```python
from build123d import *

# Parameters (mm, degrees)
SKETCH3_W               = 159.804878049
SKETCH3_H               = 120
BOSS_EXTRUDE1_DEPTH     = 10
CUT_EXTRUDE1_DEPTH      = 20
CUT_EXTRUDE3_DEPTH      = 10
CUT_EXTRUDE3_DEPTH_BACK = 16
SKETCH5_R               = 3
CUT_EXTRUDE6_DEPTH      = 10
SKETCH8_R               = 4.027386095
SKETCH8_R_2             = 4.205627654
SKETCH8_R_3             = 4.039456984
SKETCH8_R_4             = 4.036176238
BOSS_EXTRUDE3_DEPTH     = 5
SKETCH9_W               = 33.196532324
SKETCH9_H               = 25.056213838
SKETCH9_R               = 4.18060077
SKETCH9_R_2             = 4.080354001
SKETCH9_R_3             = 4.086165431
SKETCH9_R_4             = 4.036615778
BOSS_EXTRUDE4_DEPTH     = 5


with BuildPart() as part:
    # Sketch3 → Boss-Extrude1 (new body)
    with BuildSketch(Plane(origin=(0, 0, 0), x_dir=(1, 0, 0), z_dir=(0, 1, 0))):
        with Locations((34.390243903, -22.243902439)):
            Rectangle(SKETCH3_W, SKETCH3_H)
    extrude(amount=BOSS_EXTRUDE1_DEPTH)

    # Sketch4 → Cut-Extrude1 (cut)
    with BuildSketch(Plane(origin=(0, 10, 0), x_dir=(1, 0, 0), z_dir=(0, 1, 0))):
        Polygon((52.048199058, -16.00595694), (52.048199058, -34.721676718), (24.165287655, -34.721676718), (24.165287655, -6.031004918), (52.048199058, -6.031004918), align=None)
    extrude(amount=-CUT_EXTRUDE1_DEPTH, mode=Mode.SUBTRACT)

    # Sketch5 → Cut-Extrude3 (cut, two sides: drawn at the far end of the back side and taken through both)
    with BuildSketch(Plane(origin=(0, 10, 0), x_dir=(1, 0, 0), z_dir=(0, 1, 0)).offset(-CUT_EXTRUDE3_DEPTH_BACK)):
        with Locations(Location((-15.512195122, -22.243902439, 0), (0, 0, 270))):
            Circle(SKETCH5_R)
        with Locations(Location((84.292682927, -22.243902439, 0), (0, 0, 270))):
            Circle(SKETCH5_R)
    extrude(amount=CUT_EXTRUDE3_DEPTH + CUT_EXTRUDE3_DEPTH_BACK, mode=Mode.SUBTRACT)

    # Sketch7 → Cut-Extrude6 (cut)
    with BuildSketch(Plane(origin=(0, 10, 0), x_dir=(1, 0, 0), z_dir=(0, 1, 0))):
        Polygon((-6.403519992, -33.196532324), (0, -33.196532324), (0, 0), (-6.403519992, 0), (-28.646264147, 0), (-28.646264147, -33.196532324), align=None)
        Polygon((70.689603866, -33.196532324), (77.304662661, -33.196532324), (99.548678473, -33.196532324), (99.548678473, 0), (77.304662661, 0), (70.689603866, 0), align=None)
    extrude(amount=-CUT_EXTRUDE6_DEPTH, mode=Mode.SUBTRACT)

    # Sketch8 → Boss-Extrude3 (add)
    with BuildSketch(Plane.ZY):
        Polygon((0, 0), (0, 25.089225982), (33.196532324, 25.089225982), (33.196532324, 22.465752332), (33.196532324, 0), align=None)
        with Locations((4.999328758, 20.009772327)):
            Circle(SKETCH8_R, mode=Mode.SUBTRACT)
        with Locations((27.400871365, 20.009772327)):
            Circle(SKETCH8_R_2, mode=Mode.SUBTRACT)
        with Locations((4.999328758, 4.193672126)):
            Circle(SKETCH8_R_3, mode=Mode.SUBTRACT)
        with Locations((27.400871365, 4.193672126)):
            Circle(SKETCH8_R_4, mode=Mode.SUBTRACT)
    extrude(amount=BOSS_EXTRUDE3_DEPTH)

    # Sketch9 → Boss-Extrude4 (add)
    with BuildSketch(Plane(origin=(70.689603866, 0, 0), x_dir=(0, 0, -1), z_dir=(1, 0, 0))):
        with Locations((-16.598266162, 12.528106919)):
            Rectangle(SKETCH9_W, SKETCH9_H)
        with Locations((-28.524013472, 19.041369902)):
            Circle(SKETCH9_R, mode=Mode.SUBTRACT)
        with Locations((-4.413648361, 19.041369902)):
            Circle(SKETCH9_R_2, mode=Mode.SUBTRACT)
        with Locations((-28.524013472, 4.530421359)):
            Circle(SKETCH9_R_3, mode=Mode.SUBTRACT)
        with Locations((-4.413648361, 4.530421359)):
            Circle(SKETCH9_R_4, mode=Mode.SUBTRACT)
    extrude(amount=BOSS_EXTRUDE4_DEPTH)


solid = part.part
```
Can you work these out from the model? Positions are in its coordinate system, mm. A direction names the side the tool comes from. Coordinates: 2 decimals unless noted, no trailing zeros. Order: outer loops, then holes, each group sorted by start corner. A loop starts at its lowest first (then second) coordinate and runs counter-clockwise, first axis right, second up.
1. Thinking about a two-plate mould opening in Z: for faces 1 (the face through (-45.512, 5, 23)), 2 (the face through (33, 5, -37.756)), 3 (the face through (-28.646, 5, 16)), which applies, +Z half, -Z half, draft (parallel to the pull), parting line (faces both ways), or undercut?
2. If we section it at D-D (z = 55.5): Please give me the cut outline in (x, y).
3. If we section it at B-B (z = 13): Please give me the cut outline in (x, y).
4. I need wall thicknesses on line 1 (X direction, y = 2.5, z = 21); line 2 (Z direction, x = 97, y = 7.5); line 3 (X direction, y = 14.25, z = 3.5). Which ranges of each line are inside material? Lowest first, please.
5. If we section it at C-C (y = 12): Please give me the cut outline in (x, z), then the cut area to 3 significant figures.
6. For faces 4 (the face through (-2.465, 1.738, 24.198)), 5 (the face through (-2, 17, 33.197)), 6 (the face through (24.165, 5, 21)), 7 (the face through (73.155, 23.087, 4.945)), which set-ups out of +Z, -Z, +X, -X, +Y, -Y let a thin tool reach every point of the face, with its end or its side?
7. If we section it at A-A (x = 27): Please give me the cut outline in (y, z), then the cut area to 3 significant figures.
8. I'm going to push flat-ended pins straight in: pin 1 (5 mm diameter, centred on x = 98, z = 16.5, fed in from +Y); pin 2 (10.5 mm diameter, centred on y = 19.04, z = 4.41, fed in from +X); pin 3 (4 mm diameter, centred on x = 72.5, y = 20.5, fed in from -Z). Where does each tip first touch, or does it pass through?
Entries:
1. face 1: draft
1. face 2: -Z half
1. face 3: undercut
2. outline: (-45.51, 0) - (114.29, 0) - (114.29, 10) - (-45.51, 10) - close
3. outline: (-45.51, 0) - (-28.65, 0) - (-28.65, 10) - (-45.51, 10) - close; (-5, 0) - (24.17, 0) - (24.17, 10) - (0, 10) - (0, 25.09) - (-5, 25.09) - close; (52.05, 0) - (75.69, 0) - (75.69, 25.06) - (70.69, 25.06) - (70.69, 10) - (52.05, 10) - close; (99.55, 0) - (114.29, 0) - (114.29, 10) - (99.55, 10) - close
4. line 1: x = -45.51 to -28.65, -5 to 24.17, 52.05 to 75.69, 99.55 to 114.29
4. line 2: z = -37.76 to 0, 33.2 to 82.24
4. line 3: x = -5 to 0, 70.69 to 75.69
5. outline: (-5, 0) - (0, 0) - (0, 33.2) - (-5, 33.2) - close; (70.69, 0) - (75.69, 0) - (75.69, 33.2) - (70.69, 33.2) - close
5. area: 332 mm2
6. face 4: none
6. face 5: +Z, +X, -X, +Y
6. face 6: +Y, -Y
6. face 7: +X
7. outline: (0, -37.76) - (10, -37.76) - (10, 6.03) - (0, 6.03) - close; (0, 34.72) - (10, 34.72) - (10, 82.24) - (0, 82.24) - close
7. area: 913 mm2
8. pin 1: stops at y = 10
8. pin 2: stops at x = 75.69
8. pin 3: stops at z = 0
